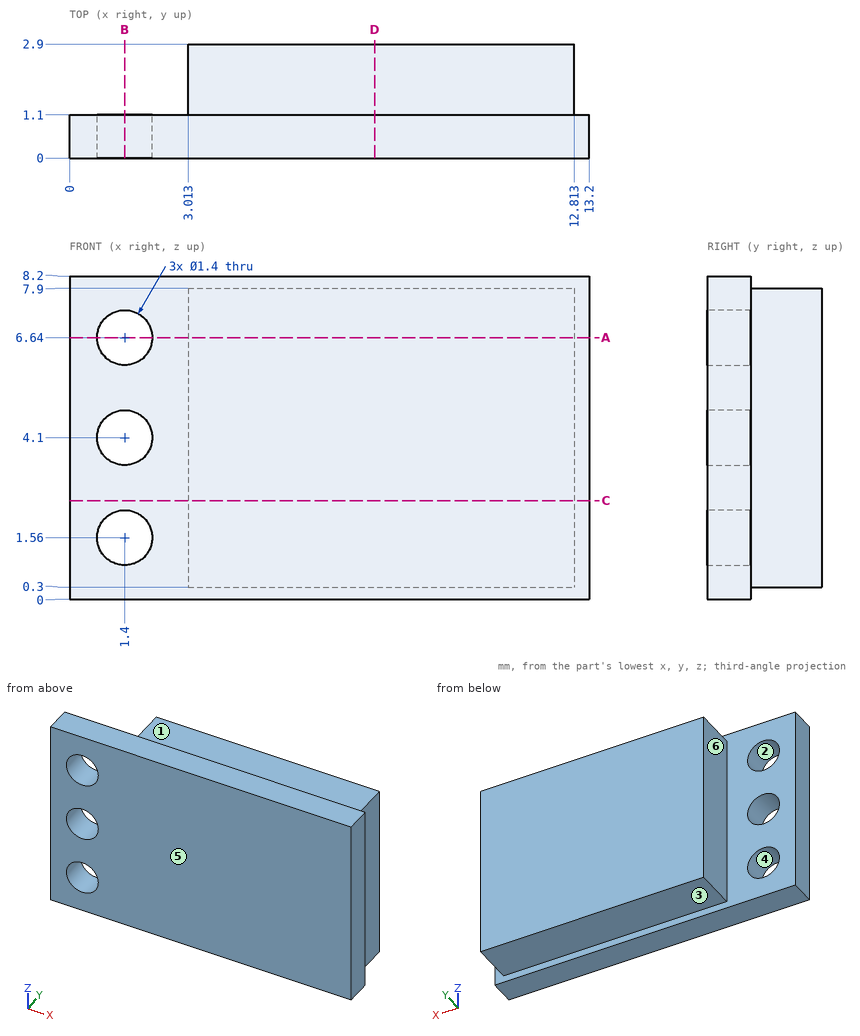
Input: dimensioned drawing with shaded views. Units: mm. Origin: part minimum x, y, z. A direction names the side the tool comes from. Coordinates: 2 decimals unless noted, no trailing zeros. Write each loop counter-clockwise with the first axis right and the second up, starting at its lowest first coordinate (ties: lowest second). Pieces come first, ordered by that corner, then holes. Notation, with made-up numbers: M 78,55.25 L 134,55.25 A13 cw 134,60.25 Z; hole C -12,-30 d5. An arc over 180 degrees is marked long. Answer as a JSON object with one key per item and string values. Group by question number.
(1) Section C-C on z = 2.5. Output: boundary loops of the cut face in (x, y).
(2) Section A-A on z = 6.64. Output: boundary loops of the cut face in (x, y), plus the area to 3 significant figures.
(3) Contact query for flat-ended pins moving along their axis: P1, Ø0.9, axis at x = 10, y = 2.5, coming from the +Z side; P2, Ø1.4, axis at x = 7, y = 2, coming from the -Z side; P3, Ø1.1, axis at x = 1.4, z = 4.1, coming from the +Y side; P4, Ø1.4, axis at y = 2, z = 5, coming from the -X side. Output: stop coordinate, or through.
(4) Ray query, line 1 along X through (y, z) = (0.5, 6.64); line 2 along X through (y, z) = (2.1, 1.25); line 3 along Y through (x, z) = (2.25, 3). Return the intervals inside material, ascending. Write a range as [from, to].
(5) Mould query, pull axis X, two halves, no side actions, for the marked faces 4, 5 and 6. Classes: pulls with the +X half, pulls with the -X half, needs draft (parallel to the pull), parting line crosses it, or undercut.
(6) Set-up query: the marked faces 1, 2 and 3. Return all of +Z, -Z, +X, -X, +Y, -Y with unobstructed straight access to the full face (end or side cutting, diameter ignored); none if empty.
(7) Section D-D on x = 7.75. Output: boundary loops of the cut face in (y, z).
(8) Section B-B on x = 1.4. Output: boundary loops of the cut face in (y, z).
Result set:
{
 "1": {"outline": "M 0,0 L 13.2,0 L 13.2,1.1 L 12.81,1.1 L 12.81,2.9 L 3.01,2.9 L 3.01,1.1 L 0,1.1 Z"},
 "2": {"outline": "M 0,0 L 0.7,0 L 0.7,1.1 L 0,1.1 Z; M 2.1,0 L 13.2,0 L 13.2,1.1 L 12.81,1.1 L 12.81,2.9 L 3.01,2.9 L 3.01,1.1 L 2.1,1.1 Z", "area": "30.6 mm2"},
 "3": {"P1": "stops at z = 7.9", "P2": "stops at z = 0.3", "P3": "passes through", "P4": "stops at x = 3.01"},
 "4": {"line 1": "x = [0, 0.7], [2.1, 13.2]", "line 2": "x = [3.01, 12.81]", "line 3": "y = [0, 1.1]"},
 "5": {"face 4": "undercut", "face 5": "needs draft", "face 6": "pulls with the -X half"},
 "6": {"face 1": "+Z, +X, -X, +Y", "face 2": "+Y, -Y", "face 3": "-Z, +X, -X, +Y"},
 "7": {"outline": "M 0,0 L 1.1,0 L 1.1,0.3 L 2.9,0.3 L 2.9,7.9 L 1.1,7.9 L 1.1,8.2 L 0,8.2 Z"},
 "8": {"outline": "M 0,0 L 1.1,0 L 1.1,0.86 L 0,0.86 Z; M 0,2.26 L 1.1,2.26 L 1.1,3.4 L 0,3.4 Z; M 0,4.8 L 1.1,4.8 L 1.1,5.94 L 0,5.94 Z; M 0,7.34 L 1.1,7.34 L 1.1,8.2 L 0,8.2 Z"}
}
